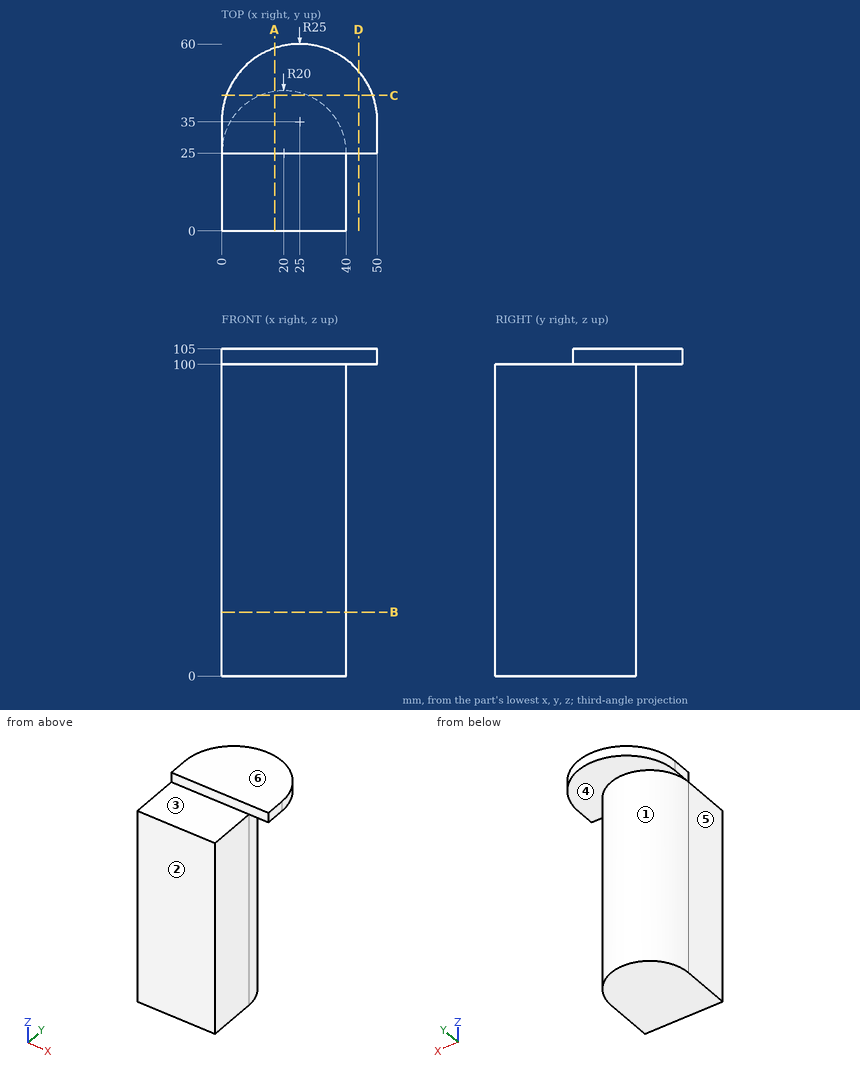
Study the drawing (mm; zero at the part's minimum x, y, z) and answer. A direction names the side the tool comes from. Coordinates: 2 decimals unless noted, no trailing zeros. Loops run counter-clockwise (first coordinate to the right, second up) from the corner with the lowest first, then second, coordinate; pieces in that order, holes last. Notation, with made-up numbers: M 5.25,36.5 L 27.25,36.5 A23 ccw 27.25,61.5 Z; hole C 38.5,-23.75 d3. An arc over 180 degrees is marked long. Answer in a Markdown table with one row per item. Add a question column.
1. Find section C-C, the plane y = 43.5. Write down the section's boundary in (x, z), then the cut area to 3 significant figures.
2. Find section D-D, the plane x = 44. Write down the section's boundary in (y, z).
3. Flat-ended cylindrical pins translate along their axes: P1, Ø4, axis at x = 14, z = 102.5, coming from the -Y side; P2, Ø5, axis at x = 27.5, y = 50.5, coming from the -Z side; P3, Ø5, axis at x = 19, y = 9.5, coming from the +Z side; P4, Ø17.5, axis at x = 30.5, y = 45.5, coming from the -Z side. Find the tip coordinate at first contact, or state that the pin passes through.
4. The mould has two halves that part along Z. Classify the marked faces 4, 5 and 6: pulls with the +Z half, pulls with the -Z half, needs draft (parallel to the pull), parting line crosses it, or undercut.
5. A tool of negligible diameter and unlimited length cuts with its end or side. For the marked faces 1, 2 and 3, from which of +Z, -Z, +X, -X, +Y, -Y can it reach the whole face along a straight path? Write none if from no direction.
6. Consider L1, parallel to X at y = 12, z = 71.5; L2, parallel to Z at x = 28, y = 6.5; L3, parallel to Z at x = 16, y = 54. Determine where each line is inside the solid, lowest interval first.
7. Find section A-A, the plane x = 17. Write down the section's boundary in (y, z), then the cut area to 3 significant figures.
8. Find section B-B, the plane z = 20.5. Write down the section's boundary in (x, y), then the cut area to 3 significant figures.
Reported:
| question | item | result |
|---|---|---|
| 1 | outline | M 1.49,100 L 12.4,100 L 12.4,0 L 27.6,0 L 27.6,100 L 48.51,100 L 48.51,105 L 1.49,105 Z |
| 1 | area | 1,750 mm^2 |
| 2 | outline | M 25,100 L 51.25,100 L 51.25,105 L 25,105 Z |
| 3 | P1 | stops at y = 25 |
| 3 | P2 | stops at z = 100 |
| 3 | P3 | stops at z = 100 |
| 3 | P4 | stops at z = 0 |
| 4 | face 4 | pulls with the -Z half |
| 4 | face 5 | needs draft |
| 4 | face 6 | pulls with the +Z half |
| 5 | face 1 | -Z, +Y |
| 5 | face 2 | +Z, -Z, +X, -X, -Y |
| 5 | face 3 | +Z, +X, -X, -Y |
| 6 | L1 | x = 0 to 40 |
| 6 | L2 | z = 0 to 100 |
| 6 | L3 | z = 100 to 105 |
| 7 | outline | M 0,0 L 44.77,0 L 44.77,100 L 58.69,100 L 58.69,105 L 25,105 L 25,100 L 0,100 Z |
| 7 | area | 4,650 mm^2 |
| 8 | outline | M 0,0 L 40,0 L 40,25 A20 ccw 0,25 Z |
| 8 | area | 1,630 mm^2 |
